from build123d import *

# Parameters (mm, degrees)
F1_W     = 3
F1_H     = 147
F1_W_2   = 95
F2_DEPTH = 3
F3_DEPTH = 12.7
F4_R     = 1.25
F5_DEPTH = 101.001


with BuildPart() as f2:
    # F1 (on Top) → F2 (new body)
    with BuildSketch(Plane.XY):
        with Locations((-49, 0)):
            Rectangle(F1_W, F1_H)
        Rectangle(F1_W_2, F1_H)
        with Locations((49, 0)):
            Rectangle(F1_W, F1_H)
    extrude(amount=F2_DEPTH)

    # F1 (on Top) → F3 (join)
    with BuildSketch(Plane.XY):
        with Locations((-49, 0)):
            Rectangle(F1_W, F1_H)
        with Locations((49, 0)):
            Rectangle(F1_W, F1_H)
    extrude(amount=F3_DEPTH)

    # F4 (on face) → F5 (cut, through all)
    with BuildSketch(Plane(origin=(-50.5, 0, 0), x_dir=(0, -1, 0), z_dir=(-1, 0, 0))):
        with Locations((-45, 6.35)):
            Circle(F4_R)
        with Locations((56.6, 6.35)):
            Circle(F4_R)
    extrude(amount=-F5_DEPTH, mode=Mode.SUBTRACT)


solid = f2.part
Read the model definition and answer for the solid it produces. Units are mm, in the model's axes. A direction names the side the tool comes from. Coordinates: 2 decimals unless noted, no trailing zeros. Write each loop counter-clockwise with the first axis right and the second up, starting at its lowest first coordinate (ties: lowest second). Pieces come first, ordered by that corner, then holes. Notation, with made-up numbers: M 70.25,-22.75 L 125.25,-22.75 A29 ccw 125.25,14.25 Z; hole C 69.25,52 d9. An arc over 180 degrees is marked long. Use a Markdown table: item, result.
Q1. Straight lines are drawn through the part: L1, parallel to X at y = 61, z = 7.5; L2, parallel to Z at x = 48.4, y = -56.6; L3, parallel to Z at x = -45, y = -3. For each, find the intervals that lie inside material, in ascending order. Write a range as [from, to].
Answer block:
| item | result |
|---|---|
| L1 | x = [-50.5, -47.5], [47.5, 50.5] |
| L2 | z = [0, 5.1], [7.6, 12.7] |
| L3 | z = [0, 3] |
Q2. The part is cut by section A-A, the plane y = 23. Write down the section's boundary in (x, z), then the cut area to 3 significant figures.
Answer block:
| item | result |
|---|---|
| outline | M -50.5,0 L 50.5,0 L 50.5,12.7 L 47.5,12.7 L 47.5,3 L -47.5,3 L -47.5,12.7 L -50.5,12.7 Z |
| area | 361 mm2 |
Q3. Each of these flat-tipped pins is pushed along its axis until it touches: pin 1 Ø2 at (y, z) = (45, 6.35) entering from +X; pin 2 Ø1 at (x, y) = (19.5, 26.5) entering from +Z. Where does it stop, or does it pass through?
Answer block:
| item | result |
|---|---|
| pin 1 | passes through |
| pin 2 | stops at z = 3 |
Q4. Determine the mould class of faces 3 (the face through (-1, 1, 3)), 4 (the face through (50.5, -1, 6)), 5 (the face through (-1, 1, 0)) for opening direction X: released by +X, released by -X, zero draft, split by the parting line, or undercut.
Answer block:
| item | result |
|---|---|
| face 3 | undercut |
| face 4 | released by +X |
| face 5 | zero draft |
Q5. The part is cut by section B-B, the plane x = -32.5. Write down the section's boundary in (y, z), then the cut area to 3 significant figures.
Answer block:
| item | result |
|---|---|
| outline | M -73.5,0 L 73.5,0 L 73.5,3 L -73.5,3 Z |
| area | 441 mm2 |
Q6. Which of the six approach directions +Z, -Z, +X, -X, +Y, -Y give full straight-line access (tool end or side, diameter ignored) to faces 1 (the face through (49, 1, 12.7)), 2 (the face through (47.5, -1, 8))?
Answer block:
| item | result |
|---|---|
| face 1 | +Z, +X, -X, +Y, -Y |
| face 2 | +Z, +Y, -Y |
